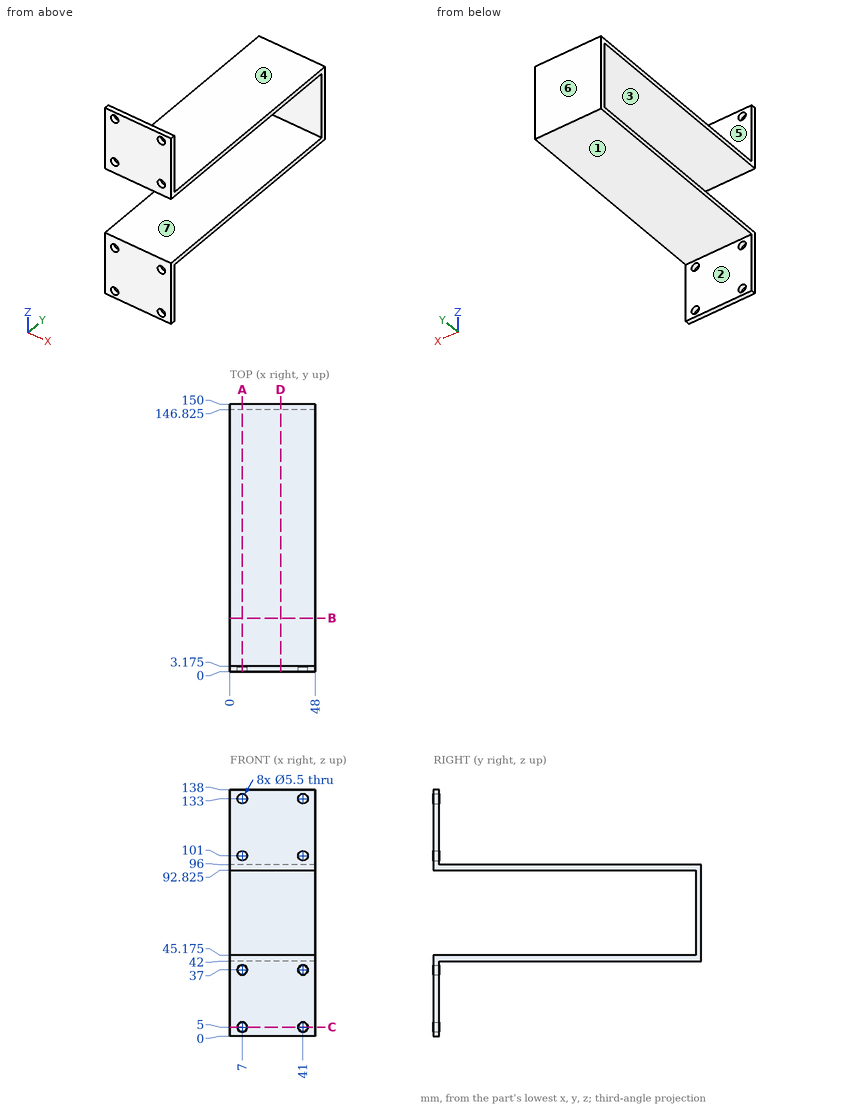
Job drawing, mm, ordinate dimensions from the low corner. One solid piece. A direction names the side the tool comes from. Coordinates: 2 decimals unless noted, no trailing zeros. Write each loop counter-clockwise with the first axis right and the second up, starting at its lowest first coordinate (ties: lowest second). Pieces come first, ordered by that corner, then holes. Notation, with made-up numbers: M 76.25,51.25 L 103.25,51.25 A12 cw 103.25,65.25 Z; hole C 26,35.5 d1. An arc over 180 degrees is marked long. Answer as a JSON object with one key per item and string values. Group by question number.
1) Saw through at A-A (x = 7). Write the cut outline in (y, z) (3 decimals).
2) Tool access for the marked faces 5, 6 and 7: list every direction of +Z, -Z, +X, -X, +Y, -Y with a clear straight run to the whole face (end or side of a thin tool).
3) Mould opens along Z. For the marked faces 1, 2, 3 and 4 say: +Z half, -Z half, draft (parallel to the pull), parting line (faces both ways), or undercut.
4) Pin check, flat tips, straight feed: pin 1 Ø12 at (x, z) = (13.5, 107) entering from +Y (3 decimals); pin 2 Ø1.5 at (x, y) = (32.5, 22.5) entering from +Z; pin 3 Ø5 at (x, z) = (41, 37) entering from -Y; pin 4 Ø1 at (x, z) = (31.5, 70) entering from -Y (3 decimals). Stop position of each tip, or through.
5) Saw through at B-B (y = 30). Write the cut outline in (x, z) (3 decimals), plus the area to 3 significant figures.
6) Saw through at C-C (z = 5). Write the cut outline in (x, y) (3 decimals), plus the area to 3 significant figures.
7) Wall check: line 1 (X direction, y = 1, z = 101); line 2 (Z direction, x = 41, y = 0.7) (3 decimals); line 3 (Z direction, x = 11.5, y = 80.5) (3 decimals). Give the ranges that are in metal, low to high. Write a range as from..to.
8) Saw through at D-D (x = 28.5). Write the cut outline in (y, z) (3 decimals), plus the area to 3 significant figures.
Values follow:
{
 "1": {"outline": "M 0,0 L 3.175,0 L 3.175,2.25 L 0,2.25 Z; M 0,7.75 L 3.175,7.75 L 3.175,34.25 L 0,34.25 Z; M 0,39.75 L 3.175,39.75 L 3.175,42 L 150,42 L 150,96 L 3.175,96 L 3.175,98.25 L 0,98.25 L 0,92.825 L 146.825,92.825 L 146.825,45.175 L 0,45.175 Z; M 0,103.75 L 3.175,103.75 L 3.175,130.25 L 0,130.25 Z; M 0,135.75 L 3.175,135.75 L 3.175,138 L 0,138 Z"},
 "2": {"face 5": "+Z, +X, -X, +Y", "face 6": "+Z, -Z, +X, -X, +Y", "face 7": "+X, -X, -Y"},
 "3": {"face 1": "-Z half", "face 2": "draft", "face 3": "undercut", "face 4": "+Z half"},
 "4": {"pin 1": "stops at y = 3.175", "pin 2": "stops at z = 96", "pin 3": "passes through", "pin 4": "stops at y = 146.825"},
 "5": {"outline": "M 0,42 L 48,42 L 48,45.175 L 0,45.175 Z; M 0,92.825 L 48,92.825 L 48,96 L 0,96 Z", "area": "305 mm2"},
 "6": {"outline": "M 0,0 L 4.25,0 L 4.25,3.175 L 0,3.175 Z; M 9.75,0 L 38.25,0 L 38.25,3.175 L 9.75,3.175 Z; M 43.75,0 L 48,0 L 48,3.175 L 43.75,3.175 Z", "area": "117 mm2"},
 "7": {"line 1": "x = 0..4.25, 9.75..38.25, 43.75..48", "line 2": "z = 0..2.25, 7.75..34.25, 39.75..45.175, 92.825..98.25, 103.75..130.25, 135.75..138", "line 3": "z = 42..45.175, 92.825..96"},
 "8": {"outline": "M 0,0 L 3.175,0 L 3.175,42 L 150,42 L 150,96 L 3.175,96 L 3.175,138 L 0,138 L 0,92.825 L 146.825,92.825 L 146.825,45.175 L 0,45.175 Z", "area": "1,370 mm2"}
}
